The model under review builds one solid part; all positions refer to its coordinate system, in mm. A direction names the side the tool comes from. Round coordinates to 2 decimals unless told otherwise and drop trailing zeros. Loops run counter-clockwise (first coordinate to the right, second up) from the corner with the lowest first, then second, coordinate; pieces in that order, holes last. Notation, with made-up numbers: (-22.5, 2) -> (-11.5, 2) arc R10 cw to (-11.5, 9) -> close; hole circle Ø7 at (78, 79). An arc over 180 degrees is marked (long way). Use a Markdown table: item, result. Add a question column.
1) For faces 5 (the flat face through (-365.5, 100, 743)), 6 (the flat face through (1061.5, 100, 743)), 7 (the flat face through (181, -75.5, 825)), 8 (the flat face through (549, -91.5, 1258)), list the 3-axis set-ups (+Z, -Z, +X, -X, +Y, -Y) from which the entire face can be reached by the end or side of a thin tool; tool diameter is ignored.
2) Wall thickness on probe 1 along Z at (x, y) = (489, -40); probe 2 along X at (y, z) = (252.5, 174); probe 3 along X at (y, z) = (54.5, 727.5): over which ranges is each line inside the solid? List them lowest first.
3) Consider section D-D on z = 1362.5. Give the boundary of the cut face in (x, y).
4) Insertion check: pin 1 (8 mm diameter, centred on x = 593.5, z = 1080, fed in from -Y); pin 2 (17.5 mm diameter, centred on x = 731, z = 467, fed in from -Y); pin 3 (4 mm diameter, centred on y = -51, z = 231, fed in from -X). Each pin has a flat end and moves straight along its axis. Give the tip position at first contact, or say it passes through.
5) Consider section A-A on x = -210.5. Give the boundary of the cut face in (y, z), plus the area to 3 significant figures.
6) Mouldability with a two-part tool opening along X and no side actions: class faces 1 (the flat face through (-367.5, 100, 1449)), 2 (the flat face through (1081, 290.5, 743)), 3 (the flat face through (904, 100, 1090.25)), 4 (the flat face through (1100.5, 100, 743)) as released by +X, released by -X, zero draft, split by the parting line, or undercut.
7) Consider section C-C on x = 504.5. Give the boundary of the cut face in (y, z), plus the area to 3 significant figures.
8) Consider section B-B on z = 532. Give the boundary of the cut face in (x, y).
from build123d import *

# Parameters (mm, degrees)
F0_W      = 697
F0_H      = 195
F0_W_2    = 36
F0_W_3    = 2
F1_DEPTH  = 36
F2_W      = 39
F2_H      = 193
F3_DEPTH  = 697.5
F4_W      = 191
F4_H      = 8
F4_H_2    = 16
F5_DEPTH  = 694
F6_W      = 16
F6_H      = 193
F6_W_2    = 8
F7_DEPTH  = 689.5
F11_W     = 16
F11_H     = 332.75
F12_DEPTH = 351.5
F13_R     = 6
F14_DEPTH = 16
F15_W     = 16
F15_H     = 160.375
F16_DEPTH = 351.5
F17_R     = 6
F18_DEPTH = 16


with BuildPart() as f1:
    # F0 (on Top) → F1 (new body)
    with BuildSketch(Plane.XY):
        with Locations((19, 0)):
            Rectangle(F0_W, F0_H)
        with Locations((-347.5, 0)):
            Rectangle(F0_W_2, F0_H)
        with Locations((-366.5, 0)):
            Rectangle(F0_W_3, F0_H)
    extrude(amount=F1_DEPTH)

    # F2 (on face) → F3 (join)
    with BuildSketch(Plane.XY.offset(36)):
        with Locations((-346, 1)):
            Rectangle(F2_W, F2_H)
    extrude(amount=F3_DEPTH)

    # F4 (on face) → F5 (join, through all)
    with BuildSketch(Plane.YZ.offset(-326.5)):
        with Locations((2, 729.5)):
            Rectangle(F4_W, F4_H)
        with Locations((2, 384.75)):
            Rectangle(F4_W, F4_H_2)
    extrude(amount=F5_DEPTH)

    # F6 (on face) → F7 (join, through all)
    with BuildSketch(Plane.XY.offset(36)):
        with Locations((0, 1)):
            Rectangle(F6_W, F6_H)
        with Locations((363.5, 1)):
            Rectangle(F6_W_2, F6_H)
    extrude(amount=F7_DEPTH)

    # F8: F1 across face


with BuildPart() as f1_1:
    add(f1.part)
    add(f1.part.mirror(Plane(origin=(0.8067832183, 1.9462668028, 733.5), x_dir=(1, 0, 0), z_dir=(0, 0, 1))))

    # F9: F1 across face


with BuildPart() as f1_2:
    add(f1_1.part)
    add(f1_1.part.mirror(Plane(origin=(367.5, 0.9612205774, 733.5), x_dir=(0, 1, 0), z_dir=(1, 0, 0))))

    # F10: F1 across face


with BuildPart() as f1_3:
    add(f1_2.part)
    add(f1_2.part.mirror(Plane(origin=(367.5, 97.5, 733.5), x_dir=(-1, 0, 0), z_dir=(0, 1, 0))))

    # F11 (on face) → F12 (join, through all)
    with BuildSketch(Plane.YZ.offset(375.5)):
        with Locations((-83.5, 1260.625)):
            Rectangle(F11_W, F11_H)
    extrude(amount=F12_DEPTH)

    # F13 (on face) → F14 (join)
    with BuildSketch(Plane.XZ.offset(91.5)):
        with Locations((700, 1260.625)):
            Circle(F13_R)
    extrude(amount=F14_DEPTH)

    # F15 (on face) → F16 (join, through all)
    with BuildSketch(Plane.YZ.offset(8)):
        with Locations((-83.5, 990.0625)):
            Rectangle(F15_W, F15_H)
        with Locations((-83.5, 825.6875)):
            Rectangle(F15_W, F15_H)
    extrude(amount=F16_DEPTH)

    # F17 (on face) → F18 (join)
    with BuildSketch(Plane.XZ.offset(91.5)):
        with Locations((183.75, 990.25)):
            Circle(F17_R)
        with Locations((183.75, 825.875)):
            Circle(F17_R)
    extrude(amount=F18_DEPTH)


solid = f1_3.part
Result set:
| question | item | result |
|---|---|---|
| 1 | face 5 | -X, +Y, -Y |
| 1 | face 6 | +Y, -Y |
| 1 | face 7 | +Y |
| 1 | face 8 | -Y |
| 2 | probe 1 | 0 to 36, 376.75 to 392.75, 725.5 to 741.5, 1074.25 to 1090.25, 1431 to 1467 |
| 2 | probe 2 | -365.5 to -326.5, -8 to 8, 359.5 to 375.5, 727 to 743, 1061.5 to 1100.5 |
| 2 | probe 3 | -365.5 to 1100.5 |
| 3 | outline | (-365.5, -95.5) -> (-326.5, -95.5) -> (-326.5, 290.5) -> (-365.5, 290.5) -> close; (-8, -95.5) -> (8, -95.5) -> (8, 290.5) -> (-8, 290.5) -> close; (359.5, -95.5) -> (375.5, -95.5) -> (375.5, -91.5) -> (727, -91.5) -> (727, -95.5) -> (743, -95.5) -> (743, 290.5) -> (727, 290.5) -> (727, -75.5) -> (375.5, -75.5) -> (375.5, 290.5) -> (359.5, 290.5) -> close; (1061.5, -95.5) -> (1100.5, -95.5) -> (1100.5, 290.5) -> (1061.5, 290.5) -> close |
| 4 | pin 1 | y = -93.5 |
| 4 | pin 2 | y = -95.5 |
| 4 | pin 3 | x = -365.5 |
| 5 | outline | (-97.5, 0) -> (292.5, 0) -> (292.5, 36) -> (-97.5, 36) -> close; (-97.5, 1431) -> (292.5, 1431) -> (292.5, 1467) -> (-97.5, 1467) -> close; (-93.5, 376.75) -> (288.5, 376.75) -> (288.5, 392.75) -> (-93.5, 392.75) -> close; (-93.5, 725.5) -> (288.5, 725.5) -> (288.5, 741.5) -> (-93.5, 741.5) -> close; (-93.5, 1074.25) -> (288.5, 1074.25) -> (288.5, 1090.25) -> (-93.5, 1090.25) -> close |
| 5 | area | 46,400 mm2 |
| 6 | face 1 | released by -X |
| 6 | face 2 | zero draft |
| 6 | face 3 | undercut |
| 6 | face 4 | released by +X |
| 7 | outline | (-97.5, 0) -> (292.5, 0) -> (292.5, 36) -> (-97.5, 36) -> close; (-97.5, 1431) -> (292.5, 1431) -> (292.5, 1467) -> (-97.5, 1467) -> close; (-93.5, 376.75) -> (288.5, 376.75) -> (288.5, 392.75) -> (-93.5, 392.75) -> close; (-93.5, 725.5) -> (288.5, 725.5) -> (288.5, 741.5) -> (-93.5, 741.5) -> close; (-93.5, 1074.25) -> (288.5, 1074.25) -> (288.5, 1090.25) -> (-93.5, 1090.25) -> close; (-91.5, 1094.25) -> (-75.5, 1094.25) -> (-75.5, 1427) -> (-91.5, 1427) -> close |
| 7 | area | 51,700 mm2 |
| 8 | outline | (-365.5, -95.5) -> (-326.5, -95.5) -> (-326.5, 290.5) -> (-365.5, 290.5) -> close; (-8, -95.5) -> (8, -95.5) -> (8, 290.5) -> (-8, 290.5) -> close; (359.5, -95.5) -> (375.5, -95.5) -> (375.5, 290.5) -> (359.5, 290.5) -> close; (727, -95.5) -> (743, -95.5) -> (743, 290.5) -> (727, 290.5) -> close; (1061.5, -95.5) -> (1100.5, -95.5) -> (1100.5, 290.5) -> (1061.5, 290.5) -> close |
